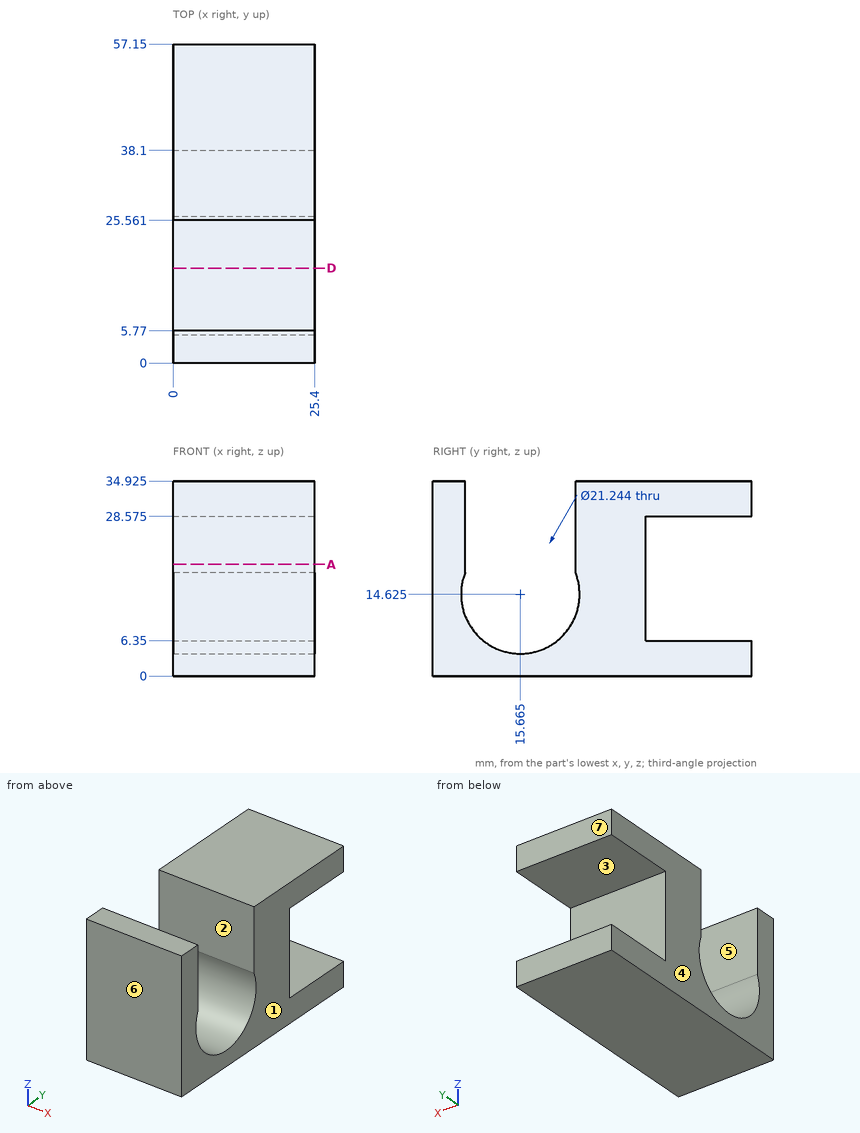
Geometry: see drawing. Coordinates: mm, zero at the bounding-box minimum. A direction names the side the tool comes from. Give positions to 0.01 mm unless a question says otherwise; leave off trailing zeros. Write each loop counter-clockwise with the first axis right and the second up, starting at its lowest first coordinate (ties: lowest second). Pieces come first, ordered by that corner, then holes. Notation, with made-up numbers: (73.25, 26) -> (92.25, 26) arc R28 ccw to (92.25, 45) -> close; hole circle Ø2 at (89, 79.25). An arc over 180 degrees is marked (long way). Use one line per item in the form item = value. Start each with the question number.
1) Set-up query: the marked faces 1, 2 and 3. Return all of +Z, -Z, +X, -X, +Y, -Y with unobstructed straight access to the full face (end or side cutting, diameter ignored); none if empty.
2) Draft query along Y for the marked faces 4, 5, 6 and 7. Return one class per face: pulls with the +Y half, pulls with the -Y half, needs draft (parallel to the pull), parting line crosses it, or undercut.
3) Section query D-D on y = 17. Return the cut outline in (x, z), then the cut area to 3 significant figures.
4) Ray query, probe 1 along Y at (x, z) = (7, 30.5); probe 2 along Y at (x, z) = (21.25, 24.5); probe 3 along Z at (x, y) = (7.75, 17). Return the intervals inside material, ascending. Write a range as from..to.
5) Pin query (flat end, axial travel): pin 1 (10 mm diameter, centred on x = 18.5, z = 20.5, fed in from +Y). Return the tip coordinate at first contact, or that it passes through.
6) Section query A-A on z = 20. Return the cut outline in (x, y).
Outcome:
q1.face_1 = +Z, -Z, +X, +Y, -Y
q1.face_2 = +Z, +X, -X
q1.face_3 = +X, -X, +Y
q2.face_4 = needs draft
q2.face_5 = undercut
q2.face_6 = pulls with the -Y half
q2.face_7 = pulls with the +Y half
q3.outline = (0, 0) -> (25.4, 0) -> (25.4, 4.09) -> (0, 4.09) -> close
q3.area = 104 mm^2
q4.probe_1 = 0..5.77, 25.56..57.15
q4.probe_2 = 0..5.77, 25.56..38.1
q4.probe_3 = 0..4.09
q5.pin_1 = 38.1
q6.outline = (0, 0) -> (25.4, 0) -> (25.4, 5.77) -> (0, 5.77) -> close; (0, 25.56) -> (25.4, 25.56) -> (25.4, 38.1) -> (0, 38.1) -> close
